The listing builds one solid part. Answer for the finished solid, in the listing's coordinates (mm). Give positions to 0.01 mm unless a question says otherwise; leave off trailing zeros. Order: outer loops, then holes, each group sorted by start corner. A loop starts at its lowest first (then second) coordinate and runs counter-clockwise, first axis right, second up.
```python
from build123d import *

# Parameters (mm, degrees)
SHELL2_T = -2


with BuildPart() as part:
    # Sketch1 → Revolve2 (revolve)
    with BuildSketch(Plane.XY, mode=Mode.PRIVATE) as revolve2_sk:
        with BuildLine():
            Line((50, 162.262364882), (13.155033794, 195))
            ThreePointArc((13.155033794, 195), (7.036599216, 198.707848685), (0, 200))
            Line((0, 200), (0, 140))
            Line((0, 140), (0, 0))
            Line((0, 0), (60, 0))
            Line((60, 0), (60, 140))
            ThreePointArc((60, 140), (57.38520841, 152.202590812), (50, 162.262364882))
        make_face()
    revolve(revolve2_sk.sketch.rotate(Axis((0, 0, 0), (0, 1, 0)), 90), axis=Axis((0, 0, 0), (0, 1, 0)))

    # Shell2
    shell2_openings = [part.faces().sort_by_distance(p)[0] for p in [
        (0, 0, 0),
    ]]
    offset(amount=SHELL2_T, openings=shell2_openings, kind=Kind.INTERSECTION)


solid = part.part
```
1) For a pull along Z with two mould halves and no side action, classify faces 1 (the cylindrical face through (51.46, 70.98, -26.76)), 2 (the cylindrical face through (-50.59, 70.98, -32.26)), 3 (the flat face through (-49.2, 0, -31.4)) as +Z half, -Z half, draft (parallel to the pull), parting line (faces both ways), or undercut.
Geometry says:
face 1: undercut
face 2: parting line
face 3: draft
2) Find section C-C (y = 101). Write down the section's boundary in (x, z).
Geometry says:
outline: circle Ø120 at (0, 0); hole circle Ø116 at (0, 0)
3) Straight lines are drawn through the part: probe 1 along X at (y, z) = (52, 0); probe 2 along Z at (x, y) = (43.5, 140.5); probe 3 along Z at (x, y) = (44, 115). For each, find the intervals that lie inside material, in ascending order.
Geometry says:
probe 1: x = -60 to -58, 58 to 60
probe 2: z = -41.32 to -38.36, 38.36 to 41.32
probe 3: z = -40.79 to -37.79, 37.79 to 40.79
4) Given P1, Ø2, axis at y = 81.5, z = -23, coming from the +X side; P2, Ø2, axis at x = -31.5, z = 18, coming from the +Y side; P3, Ø6, axis at y = 142.5, z = -9.5, coming from the -X side, each flat-ended and moving along its own axis, determine where each tip first touches the part or whether it passes through.
Geometry says:
P1: stops at x = 55.82
P2: stops at y = 175.34
P3: stops at x = -59.59
5) Find section B-B (x = 0). Write down the section's boundary in (y, z).
Geometry says:
outline: (0, -60) - (140, -60) arc R29.78 ccw to (162.26, -50) - (195, -13.16) arc R19.81 ccw to (195, 13.16) - (162.26, 50) arc R29.78 ccw to (140, 60) - (0, 60) - (0, 58) - (140, 58) arc R27.78 cw to (160.77, 48.67) - (193.5, 11.83) arc R17.81 cw to (193.5, -11.83) - (160.77, -48.67) arc R27.78 cw to (140, -58) - (0, -58) - close
6) Find section A-A (z = 0). Write down the section's boundary in (x, y).
Geometry says:
outline: (-60, 0) - (-58, 0) - (-58, 140) arc R27.78 cw to (-48.67, 160.77) - (-11.83, 193.5) arc R17.81 cw to (11.83, 193.5) - (48.67, 160.77) arc R27.78 cw to (58, 140) - (58, 0) - (60, 0) - (60, 140) arc R29.78 ccw to (50, 162.26) - (13.16, 195) arc R19.81 ccw to (-13.16, 195) - (-50, 162.26) arc R29.78 ccw to (-60, 140) - close
